from build123d import *

# Parameters (mm, degrees)
SKETCH1_W           = 65
SKETCH1_H           = 45
BOSS_EXTRUDE1_DEPTH = 3
SKETCH2_W           = 10
SKETCH2_H           = 13
BOSS_EXTRUDE2_DEPTH = 12.5
SKETCH3_R           = 1.75
CUT_EXTRUDE1_DEPTH  = 13.5
FILLET1_R           = 6
CHAMFER1_SIZE       = 12
FILLET3_R           = 1
SKETCH4_W           = 20
SKETCH4_H           = 5
CUT_EXTRUDE3_DEPTH  = 5
FILLET4_R           = 10
CHAMFER2_SIZE       = 2.5
SKETCH7_R           = 1.75
CUT_EXTRUDE4_DEPTH  = 5
BOSS_EXTRUDE4_DEPTH = 3


with BuildPart() as part:
    # Sketch1 → Boss-Extrude1 (new body)
    with BuildSketch(Plane.XY):
        with Locations((-11.936997319, -3.156836461)):
            Rectangle(SKETCH1_W, SKETCH1_H)
    extrude(amount=BOSS_EXTRUDE1_DEPTH)

    # Sketch2 → Boss-Extrude2 (add)
    with BuildSketch(Plane(origin=(0, 0, 0), x_dir=(-1, 0, 0), z_dir=(0, 0, -1))):
        with Locations((-5.563002681, -3.156836461)):
            Rectangle(SKETCH2_W, SKETCH2_H)
    extrude(amount=BOSS_EXTRUDE2_DEPTH)

    # Sketch3 → Cut-Extrude1 (cut)
    with BuildSketch(Plane(origin=(0, 3.343163539, 0), x_dir=(1, 0, 0), z_dir=(0, 1, 0))):
        with Locations(Location((5.563002681, 7.5, 0), (0, 0, 180))):
            Circle(SKETCH3_R)
    extrude(amount=-CUT_EXTRUDE1_DEPTH, mode=Mode.SUBTRACT)

    # Fillet1
    fillet1_edges = [part.edges().sort_by_distance(p)[0] for p in [
        (10.563002681, -3.156836461, -12.5),
    ]]
    fillet(fillet1_edges, radius=FILLET1_R)

    # Chamfer1
    chamfer1_edges = [part.edges().sort_by_distance(p)[0] for p in [
        (0.563002681, -3.156836461, 0),
    ]]
    chamfer(chamfer1_edges, length=CHAMFER1_SIZE)

    # Fillet3
    # the kernel refuses this fillet: 1 mm, written as the material it takes off along each edge
    with BuildSketch(Plane(origin=(0.563002681, 5.508227048, -12.5), x_dir=(1, 0, 0), z_dir=(0, -1, 0))) as fillet3_piece_1:
        with BuildLine():
            CenterArc((0.866025404, 1), FILLET3_R, 210, 60)
            Line((0, 0.5), (-0.017320508, 0.49))
            ThreePointArc((-0.017320508, 0.49), (-0.02, 0.25), (-0.02, 0))
            Line((-0.02, 0), (0, -0.02))
            Line((0, -0.02), (0.866025404, -0.02))
            Line((0.866025404, -0.02), (0.866025404, 0))
        make_face()
    extrude(amount=17.330127019, mode=Mode.SUBTRACT)

    # Sketch4 → Cut-Extrude3 (cut)
    with BuildSketch(Plane(origin=(0, 0, 0), x_dir=(-1, 0, 0), z_dir=(0, 0, -1))):
        with Locations((-5.563002681, 10.343163539)):
            Rectangle(SKETCH4_W, SKETCH4_H)
    cut_extrude3 = extrude(amount=-CUT_EXTRUDE3_DEPTH, mode=Mode.SUBTRACT)

    # Mirror2: Cut-Extrude3 across plane
    add(cut_extrude3.mirror(Plane.ZX.offset(-3.156836461)), mode=Mode.SUBTRACT)

    # Fillet4
    fillet4_edges = [part.edges().sort_by_distance(p)[0] for p in [
        (20.563002681, 19.343163539, 1.5),
        (20.563002681, -25.656836461, 1.5),
    ]]
    fillet(fillet4_edges, radius=FILLET4_R)

    # Chamfer2
    chamfer2_edges = [part.edges().sort_by_distance(p)[0] for p in [
        (10.563002681, -3.156836461, 0),
    ]]
    chamfer(chamfer2_edges, length=CHAMFER2_SIZE)

    # Sketch7 → Cut-Extrude4 (cut)
    with BuildSketch(Plane(origin=(0, 0, 0), x_dir=(-1, 0, 0), z_dir=(0, 0, -1))):
        with Locations((-17.563002681, -3.156836461)):
            Circle(SKETCH7_R)
        with Locations((-5.563002681, 16.343163539)):
            Circle(SKETCH7_R)
        with Locations((39.436997319, 16.343163539)):
            Circle(SKETCH7_R)
        with Locations(Location((39.436997319, -22.656836461, 0), (0, 0, 180))):
            Circle(SKETCH7_R)
        with Locations(Location((-5.563002681, -22.656836461, 0), (0, 0, 180))):
            Circle(SKETCH7_R)
    extrude(amount=-CUT_EXTRUDE4_DEPTH, mode=Mode.SUBTRACT)

    # Sketch8 → Boss-Extrude4 (add)
    with BuildSketch(Plane(origin=(0, 0, 0), x_dir=(-1, 0, 0), z_dir=(0, 0, -1))):
        Polygon((44.436997319, 6.843163539), (51.936997319, 6.843163539), (51.936997319, 9.343163539), (59.436997319, 4.091607002), (59.436997319, -10.405279925), (51.936997319, -15.656836461), (51.936997319, -13.156836461), (44.436997319, -13.156836461), align=None)
    extrude(amount=-BOSS_EXTRUDE4_DEPTH)


solid = part.part
Geometry: final body of the model. Coordinates: model frame, mm. A direction names the side the tool comes from. Round coordinates to 2 decimals unless told otherwise and drop trailing zeros. Loops run counter-clockwise (first coordinate to the right, second up) from the corner with the lowest first, then second, coordinate; pieces in that order, holes last. Notation, with made-up numbers: (2, -7) - (22, -7) arc R11 ccw to (22, 11) - close; hole circle Ø1 at (26, 88.5). An arc over 180 degrees is marked (long way). Write each question's results on one line, items separated by ' | '. Start each with the question number.
1) Access query for faces 4 (the face through (6, -19.157, 1)), 5 (the face through (-20, -3, 3)). Directions: +Z, -Z, +X, -X, +Y, -Y. A direction counts if a zero-diameter tool reaches every point of the face in a straight line with its end or side. Return the directions, or none.
2) Cut plane B-B on y = 0.5. Return loops of the section in (x, z).
3) Cut plane D-D on x = -49.5. Return loops of the section in (y, z).
4) Line query: probe 1 along X at (y, z) = (9, 0.25); probe 2 along Z at (x, y) = (-23, -22); probe 3 along Y at (x, z) = (14, 1.75). Output: solid intervals per line, ascending. Write a range as [from, to].
5) Mould query, pull axis X, two halves, no side actions, for faces 1 (the face through (-48, 6.843, 1)), 2 (the face through (17.56, 16.49, 1.52)), 3 (the face through (-55.634, 6.754, 1.479)). Classes: released by +X, released by -X, zero draft, split by the parting line, or undercut.
6) Cut plane C-C on x = 9. Return loops of the section in (y, z).
7) Cut plane A-A on z = -7.5. Return loops of the section in (x, y).
8) First-contact query: P1, Ø4, axis at y = -7, z = -10.5, coming from the +X side; P2, Ø2, axis at x = -17, y = 8.5, coming from the -Z side; P3, Ø4, axis at x = -5, z = -6, coming from the -Y side. Flat tips, straight axial feed; report the tip coordinate or a pass-through.
Verdict:
1) face 4: +Z, -Z | face 5: +Z, +X, -X, +Y, -Y
2) outline: (-59.44, 0) - (-11.44, 0) - (0.56, -12) arc R1 ccw to (1.43, -12.5) - (4.56, -12.5) arc R6 ccw to (10.56, -6.5) - (10.56, -2.5) - (13.06, 0) - (20.56, 0) - (20.56, 3) - (-59.44, 3) - close; hole circle Ø3.5 at (5.56, -7.5)
3) outline: (-13.16, 0) - (6.84, 0) - (6.84, 3) - (-13.16, 3) - close
4) probe 1: x = [-52.43, -51.94], [-44.44, -4.44], [15.56, 20.56] | probe 2: z = [0, 3] | probe 3: y = [-25.05, -19.16], [-14.16, 7.84], [12.84, 18.73]
5) face 1: undercut | face 2: released by +X | face 3: released by -X
6) outline: (-25.66, 0) - (-19.16, 0) - (-19.16, 3) - (-25.66, 3) - close; (-14.16, 0) - (-9.66, 0) - (-9.66, -10.54) - (3.34, -10.54) - (3.34, 0) - (7.84, 0) - (7.84, 3) - (-14.16, 3) - close; (12.84, 0) - (19.34, 0) - (19.34, 3) - (12.84, 3) - close
7) outline: (-3.94, -9.66) - (3.81, -9.66) - (3.81, 3.34) - (-3.94, 3.34) - close; (7.31, -9.66) - (10.48, -9.66) - (10.48, 3.34) - (7.31, 3.34) - close
8) P1: stops at x = 10.22 | P2: stops at z = 0 | P3: stops at y = -9.66
